Could you check a few things on this drawing? It's one solid part, dimensions in mm from its lowest x, y, z. Give positions to 0.01 mm unless a question says otherwise; leave off trailing zeros. Loops run counter-clockwise (first coordinate to the right, second up) from the corner with the lowest first, then second, coordinate; pieces in that order, holes last.
1. Imagine slicing it at B-B (x = 19.5). List the corners of the cut face in (y, z) for me, plus the area to 3 significant figures.
2. Imagine slicing it at C-C (z = 33). List the corners of the cut face in (x, y) for me (1 decimal), plus the area to 3 significant figures.
3. I need wall thicknesses on line 1 along Z through (x, y) = (32, 13) (1 decimal); line 2 along X through (y, z) = (44, 38); line 3 along X through (y, z) = (47, 13). Which ranges of each line are inside material? Lowest first, please.
4. Imagine slicing it at A-A (y = 24). List the corners of the cut face in (x, z) for me.
5. For P1, Ø6, axis at y = 41.5, z = 26, coming from the -X side; P2, Ø2, axis at x = 6, y = 16.5, coming from the +Z side (1 decimal); P3, Ø2, axis at y = 9, z = 31.5, coming from the -X side, each with a flat end and sliding along its axis, tell me the tip position at first contact or that it passes through.
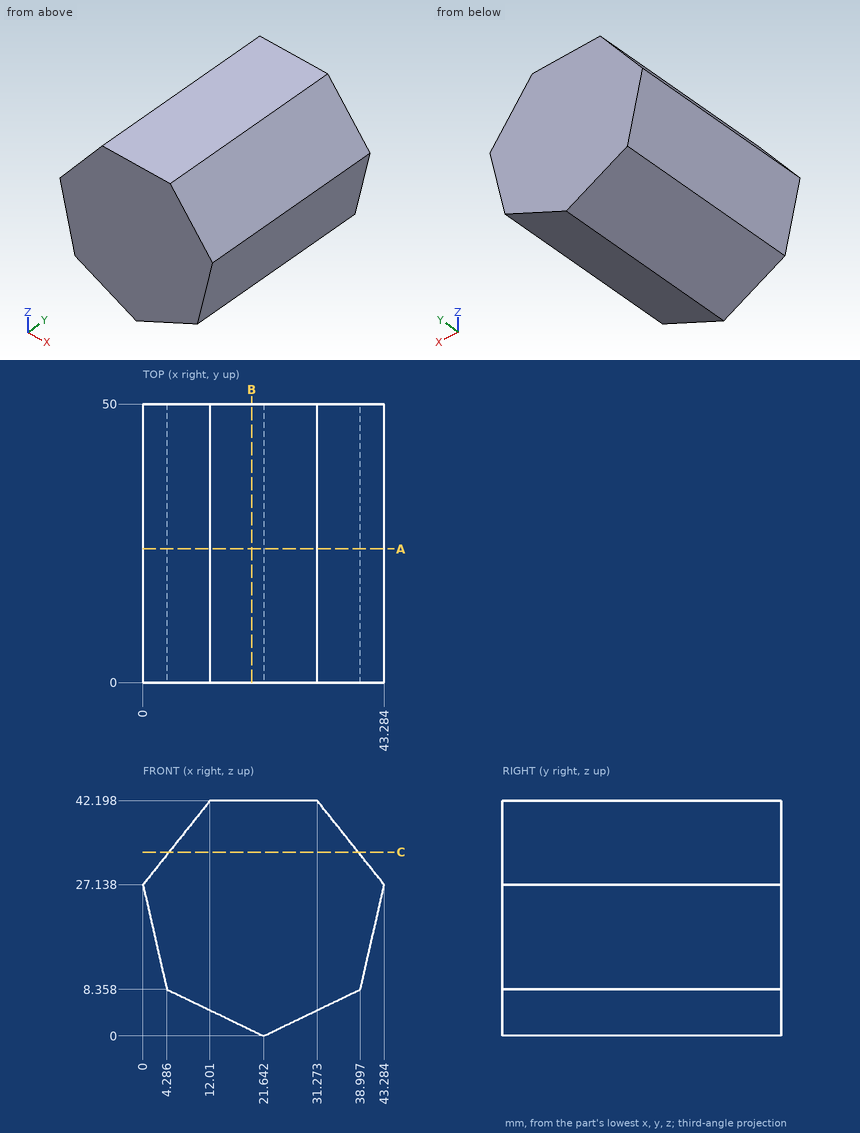
Derived:
1. outline: (0, 1.03) - (50, 1.03) - (50, 42.2) - (0, 42.2) - close
1. area: 2,060 mm2
2. outline: (4.7, 0) - (38.6, 0) - (38.6, 50) - (4.7, 50) - close
2. area: 1,700 mm2
3. line 1: z = 5 to 41.3
3. line 2: x = 8.66 to 34.62
3. line 3: x = 3.23 to 40.06
4. outline: (0, 27.14) - (4.29, 8.36) - (21.64, 0) - (39, 8.36) - (43.28, 27.14) - (31.27, 42.2) - (12.01, 42.2) - close
5. P1: stops at x = 0
5. P2: stops at z = 35.9
5. P3: stops at x = 2.68
